The listing builds one solid part. Answer for the finished solid, in the listing's coordinates (mm). Face numbers are marked on the shaded views. A direction names the side the tool comes from. Give positions to 0.01 mm unless a question says otherwise; leave off trailing zeros. Order: outer loops, then holes, each group sorted by start corner. A loop starts at its lowest first (then second) coordinate and runs counter-clockwise, first axis right, second up. Notation, with made-up numbers: (64, 3) - (85, 3) arc R32 cw to (85, 29) - close; hole circle Ø1 at (17.5, 17). An arc over 180 degrees is marked (long way). Answer in a Markdown table with one row per item.
from build123d import *

# Parameters (mm, degrees)
SKETCH1_W                 = 56
SKETCH1_H                 = 10
BOSS_EXTRUDE1_DEPTH       = 14
SKETCH9_W                 = 25
SKETCH9_H                 = 8
CUT_EXTRUDE2_DEPTH        = 5
CHAMFER2_SIZE             = 5
SKETCH10_R                = 3
CUT_EXTRUDE3_DEPTH        = 59.583274064
F_3_0MM_DOWEL_HOLE1_D     = 3.3
F_3_0MM_DOWEL_HOLE1_DEPTH = 8
F_3_0MM_DOWEL_HOLE1_TIP   = 0.991420021
FILLET1_R                 = 2


with BuildPart() as part:
    # Sketch1 → Boss-Extrude1 (new, symmetric)
    with BuildSketch(Plane.XY):
        with Locations((-28, 5)):
            Rectangle(SKETCH1_W, SKETCH1_H)
    extrude(amount=BOSS_EXTRUDE1_DEPTH, both=True)

    # Sketch9 → Cut-Extrude2 (cut)
    with BuildSketch(Plane(origin=(0, 0, 0), x_dir=(1, 0, 0), z_dir=(0, 1, 0))):
        with Locations((-31.5, 10)):
            Rectangle(SKETCH9_W, SKETCH9_H)
        with Locations((-31.5, -10)):
            Rectangle(SKETCH9_W, SKETCH9_H)
    extrude(amount=CUT_EXTRUDE2_DEPTH, mode=Mode.SUBTRACT)

    # Chamfer2
    chamfer2_edges = [part.edges().sort_by_distance(p)[0] for p in [
        (-31.5, 5, -6),
        (-31.5, 5, 6),
    ]]
    chamfer(chamfer2_edges, length=CHAMFER2_SIZE - 0.0001)  # a hair under: the kernel refuses the full size

    # Sketch10 → Cut-Extrude3 (cut, through all)
    with BuildSketch(Plane(origin=(0, 10, 0), x_dir=(1, 0, 0), z_dir=(0, 1, 0))):
        with Locations(Location((-4.5, 0, 0), (0, 0, 270))):
            Circle(SKETCH10_R)
        with Locations(Location((-13.5, 0, 0), (0, 0, 270))):
            Circle(SKETCH10_R)
        with Locations(Location((-22.5, 0, 0), (0, 0, 270))):
            Circle(SKETCH10_R)
        with Locations(Location((-31.5, 0, 0), (0, 0, 270))):
            Circle(SKETCH10_R)
    extrude(amount=-CUT_EXTRUDE3_DEPTH, mode=Mode.SUBTRACT)

    # Mirror1: part across plane


with BuildPart() as part_1:
    add(part.part)
    add(part.part.mirror(Plane(origin=(0, 10, 14), x_dir=(0, 0, 1), z_dir=(-1, 0, 0))))

    # Ø3.0mm Dowel Hole1
    with Locations(Plane(origin=(0, 10, 0), x_dir=(1, 0, 0), z_dir=(0, 1, 0))):
        with Locations((49.74, 9.5), (-49.74, -9.5), (-49.74, 9.5), (49.74, -9.5)):
            Hole(F_3_0MM_DOWEL_HOLE1_D / 2, depth=F_3_0MM_DOWEL_HOLE1_DEPTH)
            with Locations((0, 0, -(F_3_0MM_DOWEL_HOLE1_DEPTH + F_3_0MM_DOWEL_HOLE1_TIP / 2))):  # 118° drill point
                Cone(0, F_3_0MM_DOWEL_HOLE1_D / 2, F_3_0MM_DOWEL_HOLE1_TIP, mode=Mode.SUBTRACT)

    # Fillet1
    fillet1_edges = [part_1.edges().sort_by_distance(p)[0] for p in [
        (-56, 5, 14),
        (-56, 5, -14),
        (56, 5, -14),
        (56, 5, 14),
    ]]
    fillet(fillet1_edges, radius=FILLET1_R)


solid = part_1.part
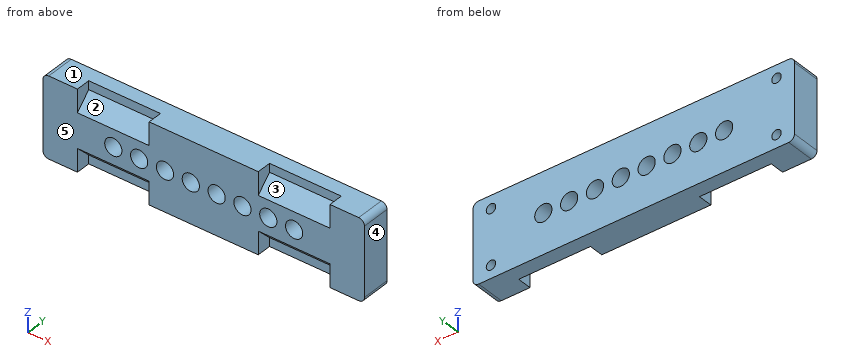
Item 1: Find section B-B on y = 9. Count the separate pieces of the cut face and the enclosed holes in it, then the cut area to 3 significant figures.
Answer block:
| item | result |
|---|---|
| separate pieces | 1 |
| enclosed holes | 12 |
| area | 2,870 mm² |
Item 2: Determine the mould class of the marked faces 3, 4 and 5 for opening direction X: pulls with the +X half, pulls with the -X half, needs draft (parallel to the pull), parting line crosses it, or undercut.
Answer block:
| item | result |
|---|---|
| face 3 | undercut |
| face 4 | pulls with the +X half |
| face 5 | needs draft |
Item 3: Consider line 1 (X direction, y = 8, z = 9.5); line 2 (X direction, y = 1.25, z = 10.25); line 3 (Z direction, x = -49.74, y = 4.5). Determine where each line is inside the solid, lowest interval first.
Answer block:
| item | result |
|---|---|
| line 1 | -56 to -51.39, -48.09 to 48.09, 51.39 to 56 |
| line 2 | -56 to -44, -19 to 19, 44 to 56 |
| line 3 | -14 to -11.15, -7.85 to 7.85, 11.15 to 14 |
Item 4: Which of the six approach directions +Z, -Z, +X, -X, +Y, -Y give full straight-line access (tool end or side, diameter ignored) to the marked faces 1 and 2?
Answer block:
| item | result |
|---|---|
| face 1 | +Z, +X, -X, +Y, -Y |
| face 2 | +Z, -Y |
Item 5: Each of these flat-tipped pins is pushed along its axis until it touches: P1, Ø1, axis at x = 3, z = 3, coming from the -Y side; P2, Ø5, axis at x = -13.5, z = 0, coming from the -Y side; P3, Ø1.5, axis at x = 31, z = 13, coming from the -Y side; P4, Ø5, axis at x = 36.5, y = 1.5, coming from the -Z side. Where does it stop, or does it pass through?
Answer block:
| item | result |
|---|---|
| P1 | y = 0 |
| P2 | through |
| P3 | y = 5 |
| P4 | z = -10 |
Item 6: Find section A-A on x = 4.5. Write down the section's boundary in (y, z).
Answer block:
| item | result |
|---|---|
| outline | (0, -14) - (10, -14) - (10, -3) - (0, -3) - close; (0, 3) - (10, 3) - (10, 14) - (0, 14) - close |
